from build123d import *

# Parameters (mm, degrees)
F0_W     = 17.873502
F0_H     = 39
F0_R     = 2
F1_DEPTH = 7
F2_W     = 17.873502
F2_H     = 39
F2_R     = 2
F2_R_2   = 4
F3_DEPTH = 3
F6_DEPTH = 1.5
F7_R     = 8


with BuildPart() as f1:
    # F0 (on Front) → F1 (new body)
    with BuildSketch(Plane.XZ):
        Rectangle(F0_W, F0_H)
        with Locations((0, -12.5)):
            Circle(F0_R, mode=Mode.SUBTRACT)
        Polygon((0, 7.505553), (6.5, 3.752777), (6.5, -3.752777), (0, -7.505553), (-6.5, -3.752777), (-6.5, 3.752777), align=None, mode=Mode.SUBTRACT)
        with Locations((0, 12.5)):
            Circle(F0_R, mode=Mode.SUBTRACT)
    extrude(amount=F1_DEPTH)

    # F2 (on face) → F3 (join)
    with BuildSketch(Plane.XZ.offset(7)):
        Rectangle(F2_W, F2_H)
        with Locations((0, -12.5)):
            Circle(F2_R, mode=Mode.SUBTRACT)
        Polygon((-6.5, -3.752777), (-6.5, 3.752777), (0, 7.505553), (6.5, 3.752777), (6.5, -3.752777), (0, -7.505553), align=None, mode=Mode.SUBTRACT)
        with Locations((0, 12.5)):
            Circle(F2_R, mode=Mode.SUBTRACT)
        Polygon((0, 7.505553), (-6.5, 3.752777), (-6.5, -3.752777), (0, -7.505553), (6.5, -3.752777), (6.5, 3.752777), align=None)
        Circle(F2_R_2, mode=Mode.SUBTRACT)
    extrude(amount=F3_DEPTH)

    # F5 (on offset) → F6 (cut, symmetric)
    with BuildSketch(Plane(origin=(0, -5, 0), x_dir=(1, 0, 0), z_dir=(0, 1, 0))):
        Polygon((3.6, -14.578461), (3.6, -10.421539), (0, -8.343078), (-3.6, -10.421539), (-3.6, -14.578461), (0, -16.656922), align=None)
        Polygon((3.6, 10.421539), (3.6, 14.578461), (0, 16.656922), (-3.6, 14.578461), (-3.6, 10.421539), (0, 8.343078), align=None)
    extrude(amount=F6_DEPTH, both=True, mode=Mode.SUBTRACT)

    # F7
    f7_edges = [f1.edges().sort_by_distance(p)[0] for p in [
        (-8.936751, -5, -19.5),
        (8.936751, -5, -19.5),
        (-8.936751, -5, 19.5),
        (8.936751, -5, 19.5),
    ]]
    fillet(f7_edges, radius=F7_R)


solid = f1.part
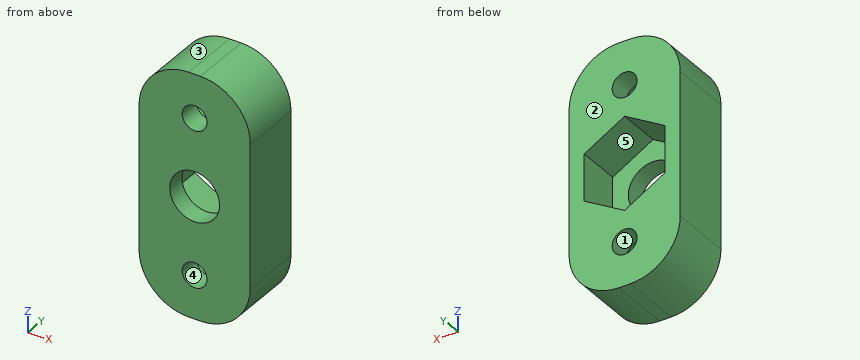
Model file for the job. Use its own axes, mm. Face numbers are marked on the shaded views. A direction names the side the tool comes from. Coordinates: 2 decimals unless noted, no trailing zeros. Order: outer loops, then holes, each group sorted by start corner. A loop starts at its lowest first (then second) coordinate and runs counter-clockwise, first axis right, second up. Notation, with made-up numbers: M 53.25,51 L 96.25,51 A17 ccw 96.25,72 Z; hole C 28,81 d4. An arc over 180 degrees is marked long. Return JSON: item names as keys, results as strings.
1. Pull direction X, two halves, no side cores. Call the marked faces 1, 2 and 3: +X half, -X half, draft (parallel to the pull), parting line (faces both ways), or undercut.
Ans:
{"face 1": "undercut", "face 2": "draft", "face 3": "-X half"}
2. Drill centre lines: probe 1 along Z at (x, y) = (0, -2.2); probe 2 along Z at (x, y) = (0, -8.9); probe 3 along Y at (x, z) = (-2.5, -11.5). Where is each one in solid material? Low to high.
Ans:
{"probe 1": "-19.5 to -14.5, -10.5 to -7.51, 7.51 to 10.5, 14.5 to 19.5", "probe 2": "-19.5 to -14.5, -10.5 to -4, 4 to 10.5, 14.5 to 19.5", "probe 3": "-10 to -6.5, -3.5 to 0"}
3. Saw through at C-C (z = 16). Give the cut face in (x, y).
Ans:
{"outline": "M -7.55,-10 L 7.55,-10 L 7.55,0 L -7.55,0 Z; hole M -1.14,-6.5 L 1.14,-6.5 L 1.14,-3.5 L -1.14,-3.5 Z"}
4. Saw through at D-D (y = -0.5). Give the cut face in (x, z).
Ans:
{"outline": "M -8.94,-11.5 A8 ccw -0.94,-19.5 L 0.94,-19.5 A8 ccw 8.94,-11.5 L 8.94,11.5 A8 ccw 0.94,19.5 L -0.94,19.5 A8 ccw -8.94,11.5 Z; hole M -6.5,-3.75 L 0,-7.51 L 6.5,-3.75 L 6.5,3.75 L 0,7.51 L -6.5,3.75 Z; hole C 0,-12.5 d4; hole C 0,12.5 d4"}
5. Tool access for the marked faces 4 and 5: list every direction of +Z, -Z, +X, -X, +Y, -Y with a clear straight run to the whole face (end or side of a thin tool).
Ans:
{"face 4": "+Y, -Y", "face 5": "+Y"}
6. Saw through at A-A (y = -5.75). Give the cut face in (x, z).
Ans:
{"outline": "M -8.94,-11.5 A8 ccw -0.94,-19.5 L 0.94,-19.5 A8 ccw 8.94,-11.5 L 8.94,11.5 A8 ccw 0.94,19.5 L -0.94,19.5 A8 ccw -8.94,11.5 Z; hole M -6.5,-3.75 L 0,-7.51 L 6.5,-3.75 L 6.5,3.75 L 0,7.51 L -6.5,3.75 Z; hole M -3.6,-14.58 L 0,-16.66 L 3.6,-14.58 L 3.6,-10.42 L 0,-8.34 L -3.6,-10.42 Z; hole M -3.6,10.42 L 0,8.34 L 3.6,10.42 L 3.6,14.58 L 0,16.66 L -3.6,14.58 Z"}
7. Flat gauge pins, fed straight in: pin 1 (1.5 mm diameter, centred on y = -4.5, z = 13.5, fed in from +X); pin 2 (2 mm diameter, centred on x = -0.5, z = -12.5, fed in from -Y); pin 3 (1.5 mm diameter, centred on y = -5, z = 13.5, fed in from -X); pin 4 (10.5 mm diameter, centred on x = 0, z = 0, fed in from +Y). Where does each tip first touch, or does it go through?
Ans:
{"pin 1": "x = 8.84", "pin 2": "through", "pin 3": "x = -8.84", "pin 4": "y = -7"}
8. Saw through at B-B (z = 0). Give the cut face in (x, y), and give its area (3 significant figures).
Ans:
{"outline": "M -8.94,-10 L -4,-10 L -4,-7 L -6.5,-7 L -6.5,0 L -8.94,0 Z; M 4,-10 L 8.94,-10 L 8.94,0 L 6.5,0 L 6.5,-7 L 4,-7 Z", "area": "63.7 mm^2"}
